Here's how the part is built. I have some questions about the finished solid (model axes, mm). Face numbers are marked on the shaded views. A direction names the side the tool comes from. Give positions to 0.01 mm unless a question says otherwise; leave off trailing zeros. Loops run counter-clockwise (first coordinate to the right, second up) from the corner with the lowest first, then second, coordinate; pieces in that order, holes last. Notation, with made-up numbers: (29.5, 43) - (85.5, 43) arc R22 cw to (85.5, 61) - close; hole circle Ø6 at (63, 33.5). An arc over 180 degrees is marked (long way). Return JSON: item names as keys, results as strings. Group by question number.
(1) On a 3-axis mill with a long thin cutter (end or side, diameter ignored), from which of +Z, -Z, +X, -X, +Y, -Y can I reach the whole of each face in a straight line? I mean the marked faces 1, 2 and 3. Say none if no direction works.
(2) If we section it at B-B (z = 10.25): Please give me the cut outline in (x, y) (3 decimals), then the cut area to 3 significant figures.
(3) If we mould it in two halves opening along Y, with no side actions, what happens to the marked faces 4, 5 and 6? For each: released by +Y, released by -Y, zero draft, split by the parting line, or undercut.
(4) For P1, Ø3.5, axis at x = 0, z = 5.5, coming from the +Y side; P2, Ø13.5, axis at x = 28.5, y = -11, coming from the +Z side; P3, Ø5, axis at x = 53.5, y = -8.5, coming from the -Z side; P4, Ø2, axis at x = -53.5, y = -7.5, coming from the +Z side, each with a flat end and sliding along its axis, tell me the tip position at first contact or that it passes through.
(5) If we section it at A-A (x = -38.5): Please give me the cut outline in (y, z), then the cut area to 3 significant figures.
(6) If we section it at C-C (x = 21): Please give me the cut outline in (y, z), then the cut area to 3 significant figures.
(7) I need wall thicknesses on probe 1 along X at (y, z) = (14.5, 4) (3 decimals); probe 2 along Y at (x, z) = (0, 11.25); probe 3 along Y at (x, z) = (-30, 7). Which ranges of each line are inside material? Lowest first, please. Write a range as [from, to].
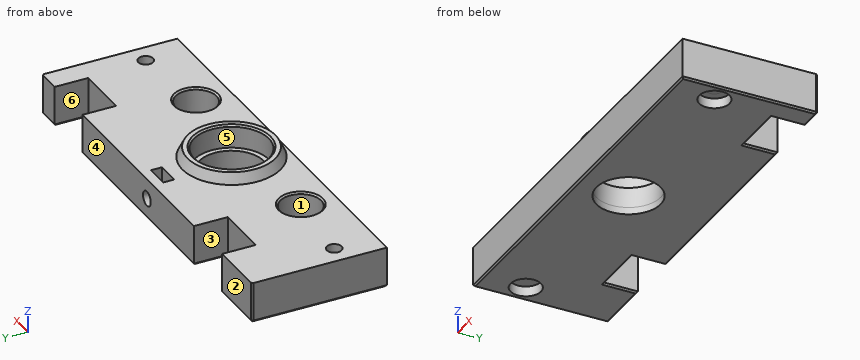
```python
from build123d import *

# Parameters (mm, degrees)
PAD005_DEPTH    = 3.3
SKETCH_W        = 120
SKETCH_H        = 40
SKETCH_R        = 6.05
SKETCH_R_2      = 2.2
SKETCH_R_3      = 11.05
PAD_DEPTH       = 12
SKETCH001_W     = 16
SKETCH001_H     = 10
POCKET_DEPTH    = 12.001
SKETCH002_R     = 4.5
POCKET001_DEPTH = 3
SKETCH003_R     = 11.05
SKETCH003_R_2   = 9.5
SKETCH003_R_3   = 6.05
PAD001_DEPTH    = 2.1
SKETCH005_R     = 11.05
SKETCH005_R_2   = 9.5
PAD002_DEPTH    = 6
SKETCH006_R     = 13
SKETCH006_R_2   = 11.05
PAD003_DEPTH    = 3
SKETCH008_R     = 2.2
POCKET002_DEPTH = 9
CHAMFER_SIZE    = 0.5
CHAMFER001_SIZE = 0.5
SKETCH004_R     = 2.2
PAD006_DEPTH    = 0.3


with BuildPart() as obj1:
    # Sketch009 → Pad005 (new body)
    with BuildSketch(Plane.XZ.offset(-17)):
        Polygon((3.525, 3.96484), (3.525, 8.03516), (3.525, 12), (-3.525, 12), (-3.525, 8.03516), (-3.525, 3.96484), (0, 1.929681), align=None)
    extrude(amount=PAD005_DEPTH)


with BuildPart() as obj2:
    # Sketch007 → Revolution (revolve)
    with BuildSketch(Plane.XZ.offset(5)):
        Polygon((13, 15), (13, 12), (14.5, 12), align=None)
    revolve(axis=Axis((0, -5, 0), (0, 0, 1)))


with BuildPart() as obj3:
    # Sketch → Pad (new body)
    with BuildSketch(Plane.XY):
        Rectangle(SKETCH_W, SKETCH_H)
        with Locations((-30, -10)):
            Circle(SKETCH_R, mode=Mode.SUBTRACT)
        with Locations((30, -10)):
            Circle(SKETCH_R, mode=Mode.SUBTRACT)
        with Locations((-54, -7.5)):
            Circle(SKETCH_R_2, mode=Mode.SUBTRACT)
        with Locations((54, -7.5)):
            Circle(SKETCH_R_2, mode=Mode.SUBTRACT)
        with Locations((0, -5)):
            Circle(SKETCH_R_3, mode=Mode.SUBTRACT)
    extrude(amount=PAD_DEPTH)

    # Sketch001 → Pocket (cut, through all)
    with BuildSketch(Plane(origin=(0, 0, 0), x_dir=(1, 0, 0), z_dir=(0, 0, -1))):
        with Locations((-35, -15)):
            Rectangle(SKETCH001_W, SKETCH001_H)
        with Locations((44.9, -15)):
            Rectangle(SKETCH001_W, SKETCH001_H)
    extrude(amount=-POCKET_DEPTH, mode=Mode.SUBTRACT)

    # Sketch002 → Pocket001 (cut)
    with BuildSketch(Plane(origin=(0, 0, 0), x_dir=(1, 0, 0), z_dir=(0, 0, -1))):
        with Locations((-54, 7.5)):
            Circle(SKETCH002_R)
        with Locations((54, 7.5)):
            Circle(SKETCH002_R)
    extrude(amount=-POCKET001_DEPTH, mode=Mode.SUBTRACT)

    # Sketch003 → Pad001 (new body)
    with BuildSketch(Plane(origin=(0, 0, 0), x_dir=(1, 0, 0), z_dir=(0, 0, -1))):
        with Locations((0, 5)):
            Circle(SKETCH003_R)
        with Locations((0, 5)):
            Circle(SKETCH003_R_2, mode=Mode.SUBTRACT)
        with Locations((-30, 10)):
            Circle(SKETCH003_R_3)
        with Locations((30, 10)):
            Circle(SKETCH003_R_3)
    extrude(amount=-PAD001_DEPTH)

    # Sketch005 → Pad002 (new body)
    with BuildSketch(Plane.XY.offset(2.1)):
        with Locations((0, -5)):
            Circle(SKETCH005_R)
        with Locations((0, -5)):
            Circle(SKETCH005_R_2, mode=Mode.SUBTRACT)
    extrude(amount=PAD002_DEPTH)

    # Sketch006 → Pad003 (new body)
    with BuildSketch(Plane.XY.offset(12)):
        with Locations((0, -5)):
            Circle(SKETCH006_R)
        with Locations((0, -5)):
            Circle(SKETCH006_R_2, mode=Mode.SUBTRACT)
    extrude(amount=PAD003_DEPTH)

    # Fusion: union obj2
    add(obj2.part)

    # Sketch008 → Pocket002 (cut)
    with BuildSketch(Plane(origin=(0, 20, 0), x_dir=(-1, 0, 0), z_dir=(0, 1, 0))):
        with Locations((0, 6)):
            Circle(SKETCH008_R)
    extrude(amount=-POCKET002_DEPTH, mode=Mode.SUBTRACT)

    # Cut: cut obj1
    add(obj1.part, mode=Mode.SUBTRACT)

    # Chamfer
    chamfer_edges = [obj3.edges().sort_by_distance(p)[0] for p in [
        (23.95, -10, 12),
        (-11.05, -5, 15),
        (-36.05, -10, 12),
    ]]
    chamfer(chamfer_edges, length=CHAMFER_SIZE)

    # Chamfer001
    chamfer001_edges = [obj3.edges().sort_by_distance(p)[0] for p in [
        (0, -20, 0),
        (60, 0, 0),
        (56.45, 20, 0),
        (52.9, 15, 0),
        (44.9, 10, 0),
        (36.9, 15, 0),
        (4.95, 20, 0),
        (-27, 15, 0),
        (-35, 10, 0),
        (-43, 15, 0),
        (-51.5, 20, 0),
        (-60, 0, 0),
        (-60, 20, 6),
        (60, 20, 6),
    ]]
    chamfer(chamfer001_edges, length=CHAMFER001_SIZE)

    # Sketch004 → Pad006 (new body)
    with BuildSketch(Plane(origin=(0, 0, 3), x_dir=(1, 0, 0), z_dir=(0, 0, -1))):
        with Locations((-54, 7.5)):
            Circle(SKETCH004_R)
        with Locations((54, 7.5)):
            Circle(SKETCH004_R)
    extrude(amount=-PAD006_DEPTH)


solid = obj3.part
```
Values:
{
 "1": {"face 1": "+Z", "face 2": "+Z, -Z, +X, -X, +Y", "face 3": "+Z, -Z, +Y"},
 "2": {"outline": "(-60, -20) - (60, -20) - (60, 19.5) - (59.5, 20) - (52.9, 20) - (52.9, 10) - (36.9, 10) - (36.9, 20) - (-27, 20) - (-27, 10) - (-43, 10) - (-43, 20) - (-59.5, 20) - (-60, 19.5) - close; hole circle Ø4.4 at (-54, -7.5); hole circle Ø12.1 at (-30, -10); hole circle Ø22.1 at (0, -5); hole (-3.525, 13.7) - (3.525, 13.7) - (3.525, 17) - (-3.525, 17) - close; hole circle Ø12.1 at (30, -10); hole circle Ø4.4 at (54, -7.5)", "area": "3,810 mm2"},
 "3": {"face 4": "released by +Y", "face 5": "undercut", "face 6": "zero draft"},
 "4": {"P1": "y = 20", "P2": "z = 12", "P3": "z = 3", "P4": "z = 3.3"},
 "5": {"outline": "(-20, 0.5) - (-19.5, 0) - (9.5, 0) - (10, 0.5) - (10, 12) - (-20, 12) - close", "area": "360 mm2"},
 "6": {"outline": "(-20, 0.5) - (-19.5, 0) - (19.5, 0) - (20, 0.5) - (20, 12) - (-20, 12) - close", "area": "480 mm2"},
 "7": {"probe 1": "[-60, -43], [-27, -3.525], [3.525, 36.9], [52.9, 60]", "probe 2": "[-20, -16.05], [6.05, 13.7], [17, 20]", "probe 3": "[-20, -16.05], [-3.95, 10]"}
}
